Answer from the drawing. Dimensions are ordinates in mm from the lowest x, y and z of the part. A direction names the side the tool comes from. Coordinates: 2 decimals unless noted, no trailing zeros. Order: outer loops, then holes, each group sorted by start corner. A loop starts at its lowest first (then second) coordinate and runs counter-clockwise, first axis right, second up. Notation, with made-up numbers: M 75.5,26 L 109.5,26 A35 ccw 109.5,59 Z; hole C -40,72 d1. An arc over 180 degrees is marked long. Write each question's results on one line, items separated by ' | '.
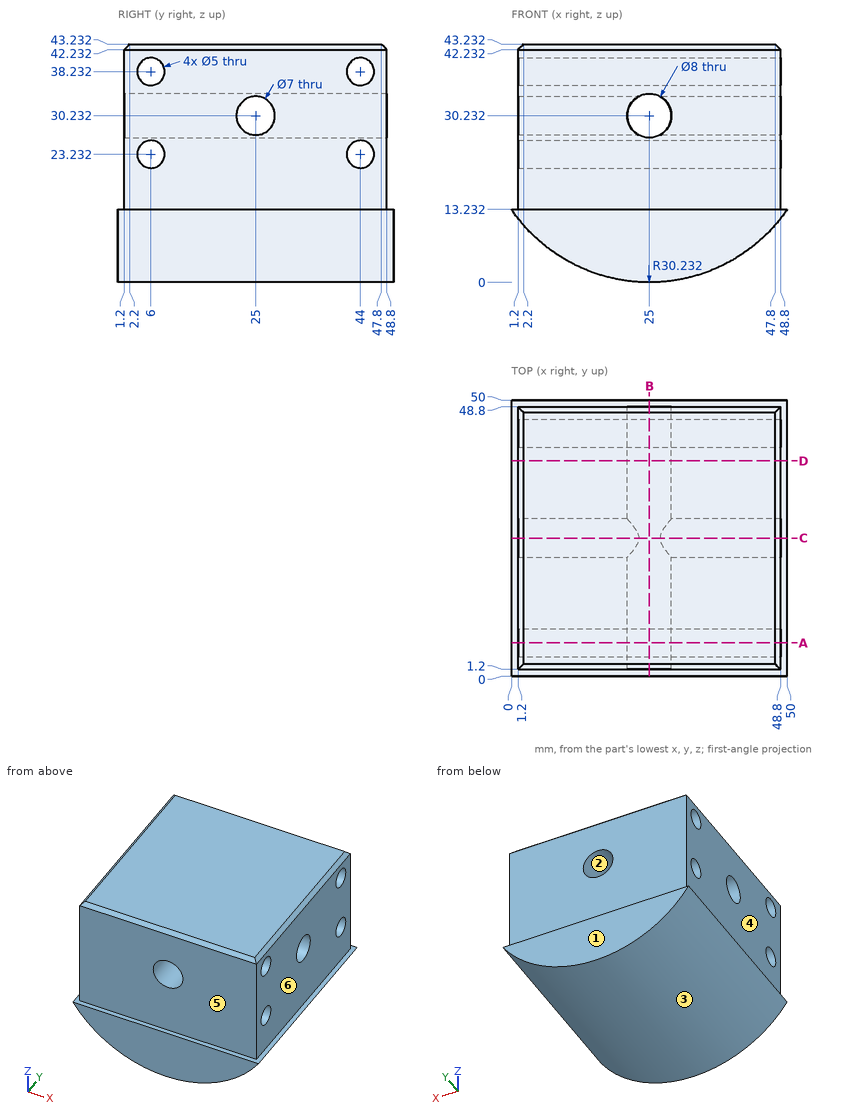
(1) The part is cut by section A-A, the plane y = 6. Write down the section's boundary in (x, z) (1 decimal).
Conclusion:
outline: M 0,13.2 A30.2 ccw 50,13.2 L 48.8,13.2 L 48.8,20.7 L 1.2,20.7 L 1.2,13.2 Z; M 1.2,25.7 L 48.8,25.7 L 48.8,35.7 L 1.2,35.7 Z; M 1.2,40.7 L 48.8,40.7 L 48.8,42.2 L 47.8,43.2 L 2.2,43.2 L 1.2,42.2 Z; hole C 25,30.2 d8
(2) For the marked faces 4, 5 and 6, determine the directions among +Z, -Z, +X, -X, +Y, -Y from which every point of the face is accessible in a straight line to the end or side of a thin tool.
Conclusion:
face 4: +Z, -X, +Y, -Y | face 5: +Z, +X, -X, -Y | face 6: +Z, +X, +Y, -Y
(3) The mould has two halves that part along X. Classify the marked faces 1, 2 and 3: pulls with the +X half, pulls with the -X half, needs draft (parallel to the pull), parting line crosses it, or undercut.
Conclusion:
face 1: needs draft | face 2: undercut | face 3: parting line crosses it
(4) The part is cut by section D-D, the plane y = 39. Write down the section's boundary in (x, z) (1 decimal).
Conclusion:
outline: M 0,13.2 A30.2 ccw 50,13.2 L 48.8,13.2 L 48.8,42.2 L 47.8,43.2 L 2.2,43.2 L 1.2,42.2 L 1.2,13.2 Z; hole C 25,30.2 d8
(5) The part is cut by section B-B, the plane x = 25. Write down the section's boundary in (y, z), then the cut area to 3 significant figures.
Conclusion:
outline: M 0,0 L 50,0 L 50,13.23 L 48.8,13.23 L 48.8,26.23 L 1.2,26.23 L 1.2,13.23 L 0,13.23 Z; M 1.2,34.23 L 48.8,34.23 L 48.8,42.23 L 47.8,43.23 L 2.2,43.23 L 1.2,42.23 Z; hole C 6,23.23 d5; hole C 6,38.23 d5; hole C 44,23.23 d5; hole C 44,38.23 d5 | area: 1,630 mm²
(6) The part is cut by section C-C, the plane y = 25. Write down the section's boundary in (x, z) (1 decimal), then the cut area to 3 significant figures.
Conclusion:
outline: M 0,13.2 A30.2 ccw 50,13.2 L 48.8,13.2 L 48.8,26.7 L 26.9,26.7 A4 cw 23.1,26.7 L 1.2,26.7 L 1.2,13.2 Z; M 1.2,33.7 L 23.1,33.7 A4 cw 26.9,33.7 L 48.8,33.7 L 48.8,42.2 L 47.8,43.2 L 2.2,43.2 L 1.2,42.2 Z | area: 1,560 mm²
(7) Given pin 1 (5 mm diameter, centred on x = 16, y = 15.5, fed in from -Z); pin 2 (3 mm diameter, centred on y = 44, z = 23.23, fed in from +X); pin 3 (6 mm diameter, centred on y = 44, z = 38.23, fed in from +X); pin 4 (23 mm diameter, centred on y = 13.5, z = 29, fed in from -X), each flat-ended and moving along its own axis, determine where each tip first touches the part or whether it passes through.
Conclusion:
pin 1: z = 0.71 | pin 2: through | pin 3: x = 48.8 | pin 4: x = 1.2
(8) Straight lines are drawn through the part: line 1 (Y direction, x = 27.5, z = 23); line 2 (Y direction, x = 16.5, z = 22) (1 decimal); line 3 (Y direction, x = 20, z = 30.5). For each, find the intervals that lie inside material, in ascending order.
Conclusion:
line 1: 1.2 to 3.51, 8.49 to 41.51, 46.49 to 48.8 | line 2: 1.2 to 3.8, 8.2 to 41.8, 46.2 to 48.8 | line 3: 1.2 to 21.51, 28.49 to 48.8
